Geometry check sheet. Reference: the model listing, model coordinates, mm. A direction names the side the tool comes from. Round coordinates to 2 decimals unless told otherwise and drop trailing zeros. Write each loop counter-clockwise with the first axis right and the second up, starting at its lowest first coordinate (ties: lowest second). Pieces come first, ordered by that corner, then holes. Notation, with made-up numbers: (71.25, 19.5) -> (122.25, 19.5) arc R14 ccw to (122.25, 29.5) -> close; hole circle Ø5 at (4.5, 80.5). An arc over 180 degrees is marked (long way). Use a Markdown table: item, result.
Autodesk Inventor part; units mm, degrees
ref_plane "YZ Plane" through (0, 0, 0) normal (1, 0, 0) x (0, 1, 0)
ref_plane "XZ Plane" through (0, 0, 0) normal (0, 1, 0) x (-1, 0, 0)
ref_plane "XY Plane" through (0, 0, 0) normal (0, 0, 1) x (1, 0, 0)
sketch "Sketch1" plane through (0, 0, 0) normal (0, 1, 0) x (-1, 0, 0)
  circle A0 centre (0, 0) radius 35
  circle A1 centre (15, 15) radius 1.6
  circle A2 centre (15, -15) radius 1.6
  circle A3 centre (-15, -15) radius 1.6
  circle A4 centre (-15, 15) radius 1.6
  line L0 (15, 15) -> (-15, 15) construction
  line L1 (-15, 15) -> (-15, -15) construction
  line L2 (-15, -15) -> (15, -15) construction
  line L3 (15, -15) -> (15, 15) construction
  circle A5 centre (0, 0) radius 10
  dimension "d1" = 30
  dimension "d2" = 30
  dimension "d4" = 3.2
  dimension "d5" = 3.2
  dimension "d6" = 3.2
  dimension "d7" = 3.2
  dimension "d8" = 15
  dimension "d9" = 15
  dimension "d10" = 20
  dimension "d11" = 70
extrude "Extrusion1" add sketch "Sketch1" along normal blind 20
sketch "Sketch2" plane through (0, 20, 0) normal (0, 1, 0) x (1, 0, 0)
  circle A0 centre (-15, -15) radius 1.6
  circle A1 centre (-15, -15) radius 2.5
  circle A2 centre (-15, 15) radius 1.6
  circle A3 centre (-15, 15) radius 2.5
  circle A4 centre (15, 15) radius 2.5
  circle A5 centre (15, -15) radius 2.5
  point P0 (0, 0)
  dimension "d14" = 15
  dimension "d15" = 15
  dimension "d16" = 15
  dimension "d17" = 15
  dimension "d18" = 5
  dimension "d19" = 5
  dimension "d20" = 5
  dimension "d21" = 5
extrude "Extrusion2" cut sketch "Sketch2" against normal blind 15
sketch "Sketch3" plane through (0, 20, 0) normal (0, 1, 0) x (1, 0, 0)
  line L0 (-12.75, -23.45) -> (-4.841, -23.45)
  line L1 (-4.841, -23.45) -> (-4.841, -17)
  line L2 (-4.841, -17) -> (-12.75, -17)
  line L3 (-12.75, -17) -> (-12.75, -23.45)
  line L4 (-1.941, -23.45) -> (7.059, -23.45)
  line L5 (7.059, -23.45) -> (7.059, -17)
  line L6 (7.059, -17) -> (-1.941, -17)
  line L7 (-1.941, -17) -> (-1.941, -23.45)
  line L8 (-11.75, 17) -> (-5.841, 17)
  line L9 (-4.841, 18) -> (-4.841, 22.3739)
  line L10 (-5.8263, 23.45) -> (-11.7381, 23.45)
  line L11 (-12.7499, 22.4501) -> (-12.7499, 18)
  line L12 (-0.941, 17) -> (6.059, 17)
  line L13 (7.059, 18) -> (7.059, 22.45)
  line L14 (6.059, 23.45) -> (-0.941, 23.45)
  line L15 (-1.941, 22.45) -> (-1.941, 18)
  arc A0 (-12.7499, 18) -> (-11.75, 17) centre (-12.75, 17) ccw
  arc A1 (-11.7381, 23.45) -> (-12.7499, 22.4501) centre (-12.7381, 23.45) ccw
  arc A2 (-4.841, 22.3739) -> (-5.8263, 23.45) centre (-4.8292, 23.3739) ccw
  arc A3 (-5.841, 17) -> (-4.841, 18) centre (-4.841, 17) ccw
  arc A4 (7.059, 22.45) -> (6.059, 23.45) centre (7.059, 23.45) ccw
  arc A5 (6.059, 17) -> (7.059, 18) centre (7.059, 17) ccw
  arc A6 (-1.941, 18) -> (-0.941, 17) centre (-1.941, 17) ccw
  arc A7 (-0.941, 23.45) -> (-1.941, 22.45) centre (-1.941, 23.45) ccw
  point P0 (0, 0)
  dimension "d24" = 17
  dimension "d25" = 17
  dimension "d26" = 6.45
  dimension "d27" = 6.45
  dimension "d28" = 2.9
  dimension "d29" = 7.909
  dimension "d30" = 9
  dimension "d31" = 1.941
  dimension "d32" = 34
  dimension "d33" = 6.45
  dimension "d42" = 2
  dimension "d43" = 2
  dimension "d44" = 2
  dimension "d45" = 2
  dimension "d46" = 2
  dimension "d47" = 2
  dimension "d50" = 2
  dimension "d51" = 2
extrude "Extrusion3" cut sketch "Sketch3" against normal blind 25
sketch "Sketch5" plane through (0, 20, 0) normal (0, 1, 0) x (1, 0, 0)
  line L0 (-20, -26) -> (20, -26)
  line L1 (20, -26) -> (20, 26)
  line L2 (20, 26) -> (-20, 26)
  line L3 (-20, 26) -> (-20, -26)
  line L4 (-12.5, -12.5) -> (12.5, -12.5)
  line L5 (12.5, -12.5) -> (12.5, 12.5)
  line L6 (12.5, 12.5) -> (-12.5, 12.5)
  line L7 (-12.5, 12.5) -> (-12.5, -12.5)
  point P0 (0, 0)
  dimension "d64" = 52
  dimension "d65" = 40
  dimension "d66" = 20
  dimension "d67" = 26
  dimension "d70" = 25
  dimension "d71" = 25
  dimension "d72" = 12.5
  dimension "d73" = 12.5
extrude "Extrusion5" cut sketch "Sketch5" against normal blind 30 keep common part
fillet "Fillet1" radius 2 1 edges at (-20, 10, 26)
fillet "Fillet2" radius 2 1 edges at (20, 10, 26)
fillet "Fillet3" radius 2 1 edges at (20, 10, -26)
fillet "Fillet4" radius 2 1 edges at (-20, 10, -26)
fillet "Fillet5" radius 2 1 edges at (12.5, 10, 12.5)
fillet "Fillet6" radius 2 1 edges at (-12.5, 10, -12.5)
fillet "Fillet7" radius 2 2 edges at (12.5, 10, -12.5) (-12.5, 10, 12.5)
sketch "Sketch6" plane through (-18, 0, 26) normal (0, 0, 1) x (1, 0, 0)
  circle A0 centre (9, 7) radius 1.55
  circle A1 centre (9, 14) radius 1.55
  circle A2 centre (21, 7) radius 1.55
  circle A3 centre (21, 14) radius 1.55
  line L0 (0, 0) -> (36, 0)
  line L1 (18, 0) -> (18, 20) construction
  dimension "d81" = 3.1
  dimension "d82" = 3.1
  dimension "d83" = 3.1
  dimension "d84" = 3.1
  dimension "d85" = 7
  dimension "d86" = 7
  dimension "d87" = 7
  dimension "d88" = 7
  dimension "d89" = 0
  dimension "d90" = 3
  dimension "d91" = 3
  dimension "d92" = 9
  dimension "d93" = 9
extrude "Extrusion6" cut sketch "Sketch6" against normal blind 100
sketch "Sketch7" plane through (0, 20, 0) normal (0, 1, 0) x (1, 0, 0)
  circle A0 centre (-15, -15) radius 2.5
  circle A1 centre (-12.75, -23.45) radius 1
  circle A2 centre (-4.8235, -23.45) radius 1
  circle A3 centre (-4.841, -17) radius 1
  circle A4 centre (-1.941, -17) radius 1
  circle A5 centre (-1.941, -23.45) radius 1
  circle A6 centre (7.0924, -17) radius 1
  circle A7 centre (7.0924, -23.45) radius 1
  circle A8 centre (-12.75, -17) radius 1
  point P0 (0, 0)
  dimension "d96" = 2
  dimension "d97" = 2
  dimension "d98" = 2
  dimension "d99" = 2
  dimension "d100" = 2
  dimension "d101" = 2
  dimension "d102" = 2
  dimension "d103" = 2
extrude "Extrusion7" cut sketch "Sketch7" against normal blind 100 contours A8 A0 | A0 A8 | A1 | A2 | A3 | A4 | A5 | A6 | A7 picked at (-13.2603, -16.5464) picked at (-12.7663, -16.994)
sketch "Sketch8" plane through (0, 0, 0) normal (0, -1, 0) x (1, 0, 0)
  line L0 (15, 26) -> (20, 21)
  line L1 (20, 24) -> (20, -24)
  line L2 (15, 26) -> (20, 26)
  line L3 (20, 21) -> (20, 26)
  line L4 (-18, 26) -> (18, 26)
  line L5 (-15, 26) -> (-20, 26)
  line L6 (-20, 26) -> (-20, 21)
  line L7 (-20, 21) -> (-15, 26)
  line L8 (-20, -24) -> (-20, 24)
  line L9 (-20, -21) -> (-20, -26)
  line L10 (-20, -26) -> (-15, -26)
  line L11 (-15, -26) -> (-20, -21)
  line L12 (18, -26) -> (-18, -26)
  line L13 (20, -21) -> (20, -26)
  line L14 (20, -26) -> (15, -26)
  line L15 (20, -21) -> (15, -26)
  point P0 (0, 0)
  dimension "d106" = 5
  dimension "d107" = 5
  dimension "d108" = 5
  dimension "d109" = 5
  dimension "d110" = 5
  dimension "d111" = 5
  dimension "d112" = 5
  dimension "d113" = 5
extrude "Extrusion8" cut sketch "Sketch8" against normal blind 20 contours L2 L3 L1 L0 | L7 L6 L5 L4 | L1 L13 L14 L12 L15 | L11 L10 L9 L8
fillet "Fillet8" radius 2 1 edges at (15, 10, 26)
fillet "Fillet9" radius 2 1 edges at (20, 10, 21)
fillet "Fillet10" radius 2 1 edges at (20, 10, -21)
fillet "Fillet11" radius 2 3 edges at (15, 10, -26) (-15, 10, 26) (-20, 10, 21)
fillet "Fillet12" radius 2 2 edges at (-20, 10, -21) (-15, 10, -26)
equation "\"d5\" = d4"
equation "\"d6\" = d5"
equation "\"d7\" = d4"
equation "\"d19\" = d18"
equation "\"d20\" = d18"
equation "\"d21\" = d19"
equation "\"d27\" = d26"
equation "\"d32\" = 2 * d24"
equation "\"d33\" = d26"
equation "\"d87\" = d85"
equation "\"d88\" = d86"
properties part number "supportHolder"
(1) Thickness scan on line 1 (Z direction, x = 0, y = 18.25); line 2 (Y direction, x = -9, z = -15.6); line 3 (X direction, y = 15.25, z = -15.5). Record the ranges inside material, lowest first.
A:
| item | result |
|---|---|
| line 1 | z = -26 to -23.45, -17 to -12.5, 12.5 to 17, 23.45 to 26 |
| line 2 | y = 0 to 5.45, 8.55 to 12.45, 15.55 to 20 |
| line 3 | x = -20 to -17.45, -12.55 to -9.92, -8.08 to 2.08, 3.92 to 12.55, 17.45 to 20 |
(2) Access from +Z, -Z, +X, -X, +Y, -Y to the whole of each face (thin tool, end or side, straight path). Record for faces 5 (the face through (7.059, 10, -20)), 6 (the face through (1.77, 6.06, -14.72)).
A:
| item | result |
|---|---|
| face 5 | +Y, -Y |
| face 6 | +Z, -Z |
(3) Section check D-D on x = 3. State how many separate pieces and enclosed holes the cut face has, plus the area to 3 significant figures.
A:
| item | result |
|---|---|
| separate pieces | 12 |
| enclosed holes | 0 |
| area | 195 mm2 |
(4) Gauge pin test, flat end, axial feed: pin 1 Ø1.5 at (x, z) = (10.5, 1.5) entering from +Y. Record the tip position at first contact, or that the pin passes through.
A:
| item | result |
|---|---|
| pin 1 | passes through |
(5) Section check A-A on z = 5.5. Record the cut outline in (x, y).
A:
| item | result |
|---|---|
| outline | (-20, 0) -> (-12.5, 0) -> (-12.5, 20) -> (-20, 20) -> close; (12.5, 0) -> (20, 0) -> (20, 20) -> (12.5, 20) -> close |
(6) Section check C-C on x = 11.5. Record the cut outline in (y, z).
A:
| item | result |
|---|---|
| outline | (0, -26) -> (20, -26) -> (20, -12.23) -> (0, -12.23) -> close; (0, 12.23) -> (20, 12.23) -> (20, 26) -> (0, 26) -> close |
(7) Release check for a two-part mould opening along Y. For faces 1 (the face through (-8.285, 5.625, 14.781)), 2 (the face through (1.77, 6.06, 14.78)), 3 (the face through (14, 20, 0)), 4 (the face through (-11.93, 9.86, -11.9)) record: +Y half, -Y half, draft (parallel to the pull), parting line (faces both ways), or undercut.
A:
| item | result |
|---|---|
| face 1 | undercut |
| face 2 | undercut |
| face 3 | +Y half |
| face 4 | draft |
(8) Section check B-B on z = -15. Record the cut outline in (x, y).
A:
| item | result |
|---|---|
| outline | (-20, 0) -> (-16.6, 0) -> (-16.6, 5) -> (-17.5, 5) -> (-17.5, 20) -> (-20, 20) -> close; (-13.4, 0) -> (13.4, 0) -> (13.4, 5) -> (12.5, 5) -> (12.5, 20) -> (-12.5, 20) -> (-12.5, 5) -> (-13.4, 5) -> close; (16.6, 0) -> (20, 0) -> (20, 20) -> (17.5, 20) -> (17.5, 5) -> (16.6, 5) -> close; hole circle Ø3.1 at (-9, 7); hole circle Ø3.1 at (-9, 14); hole circle Ø3.1 at (3, 7); hole circle Ø3.1 at (3, 14) |
